Read the model definition and answer for the solid it produces. Units are mm, in the model's axes. Face numbers are marked on the shaded views. A direction names the side the tool comes from. Coordinates: 2 decimals unless noted, no trailing zeros. Loops run counter-clockwise (first coordinate to the right, second up) from the corner with the lowest first, then second, coordinate; pieces in that order, holes last. Notation, with made-up numbers: M 49,14.5 L 79,14.5 A4 cw 79,20.5 Z; hole C 22,75 d3. An arc over 180 degrees is marked long. One line per item, written item: value. Start each with the question number.
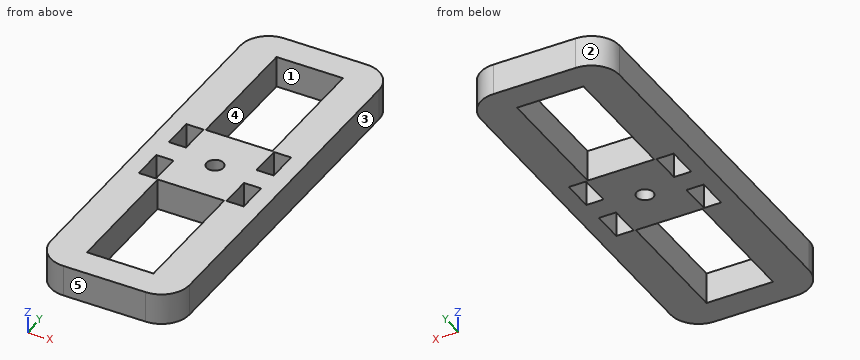
```python
from build123d import *

# Parameters (mm, degrees)
SKETCH1_W           = 3.055
SKETCH1_H           = 5.575
SKETCH1_W_2         = 11.81
SKETCH1_H_2         = 22.57
SKETCH1_R           = 1.475
BOSS_EXTRUDE1_DEPTH = 5.58


with BuildPart() as part:
    # Sketch1 → Boss-Extrude1 (new body)
    with BuildSketch(Plane.XY):
        with BuildLine():
            Line((708.390729089, 432.709671907), (715.695729089, 432.709671907))
            Line((715.695729089, 432.709671907), (723.000729089, 432.709671907))
            ThreePointArc((723.000729089, 432.709671907), (726.536262995, 434.174138001), (728.000729089, 437.709671907))
            Line((728.000729089, 437.709671907), (728.000729089, 498.199671907))
            ThreePointArc((728.000729089, 498.199671907), (726.536262995, 501.735205812), (723.000729089, 503.199671907))
            Line((723.000729089, 503.199671907), (715.695729089, 503.199671907))
            Line((715.695729089, 503.199671907), (708.390729089, 503.199671907))
            ThreePointArc((708.390729089, 503.199671907), (704.855195183, 501.735205812), (703.390729089, 498.199671907))
            Line((703.390729089, 498.199671907), (703.390729089, 437.709671907))
            ThreePointArc((703.390729089, 437.709671907), (704.855195183, 434.174138001), (708.390729089, 432.709671907))
        make_face()
        with Locations((707.918229089, 463.167171907)):
            Rectangle(SKETCH1_W, SKETCH1_H, mode=Mode.SUBTRACT)
        with Locations((715.695729089, 448.994671907)):
            Rectangle(SKETCH1_W_2, SKETCH1_H_2, mode=Mode.SUBTRACT)
        with Locations((715.695729089, 467.954671907)):
            Circle(SKETCH1_R, mode=Mode.SUBTRACT)
        with Locations((723.473229089, 463.167171907)):
            Rectangle(SKETCH1_W, SKETCH1_H, mode=Mode.SUBTRACT)
        with Locations((707.918229089, 472.742171907)):
            Rectangle(SKETCH1_W, SKETCH1_H, mode=Mode.SUBTRACT)
        with Locations((723.473229089, 472.742171907)):
            Rectangle(SKETCH1_W, SKETCH1_H, mode=Mode.SUBTRACT)
        with Locations((715.695729089, 486.914671907)):
            Rectangle(SKETCH1_W_2, SKETCH1_H_2, mode=Mode.SUBTRACT)
    extrude(amount=BOSS_EXTRUDE1_DEPTH)


solid = part.part
```
1) Flat-ended cylindrical pins translate along their axes: pin 1 (1.5 mm diameter, centred on x = 724, z = 4, fed in from -Y); pin 2 (2 mm diameter, centred on x = 719, y = 453.5, fed in from -Z); pin 3 (1.5 mm diameter, centred on x = 724.5, z = 2, fed in from +Y); pin 4 (0.9 mm diameter, centred on x = 707.5, z = 3, fed in from +Y). Find the tip coordinate at first contact, or state that the pin passes through.
2) Section C-C (x = 715) is taken. Determine the outline of the cut face in (y, z), then the cut area to 3 significant figures.
3) A tool of negligible diameter and unlimited length cuts with its end or side. For the marked faces 1 and 2, from which of +Z, -Z, +X, -X, +Y, -Y can it reach the whole face along a straight path? Write none if from no direction.
4) Consider line 1 along Y through (x, z) = (708.75, 4.1); line 2 along Y through (x, z) = (710.25, 2.05); line 3 along X through (y, z) = (472, 3.8). Determine where each line is inside the solid, lowest interval first.
5) Section B-B (y = 478) is taken. Determine the outline of the cut face in (x, z), then the cut area to 3 significant figures.
6) For a pull along Y with two mould halves and no side action, classify the marked faces 3, 4 and 5 as released by +Y, released by -Y, zero draft, split by the parting line, or undercut.
7) Section D-D (x = 718.5) is taken. Determine the outline of the cut face in (y, z).
8) Section A-A (y = 462.5) is taken. Determine the outline of the cut face in (x, z), then the cut area to 3 significant figures.
Results found:
1. pin 1: stops at y = 432.72
1. pin 2: passes through
1. pin 3: stops at y = 503.14
1. pin 4: stops at y = 503.18
2. outline: M 432.71,0 L 437.71,0 L 437.71,5.58 L 432.71,5.58 Z; M 460.28,0 L 466.65,0 L 466.65,5.58 L 460.28,5.58 Z; M 469.26,0 L 475.63,0 L 475.63,5.58 L 469.26,5.58 Z; M 498.2,0 L 503.2,0 L 503.2,5.58 L 498.2,5.58 Z
2. area: 127 mm²
3. face 1: +Z, -Z
3. face 2: +Z, -Z, -X, +Y
4. line 1: y = 432.71 to 460.38, 465.95 to 469.95, 475.53 to 503.2
4. line 2: y = 432.71 to 437.71, 460.28 to 475.63, 498.2 to 503.2
4. line 3: x = 703.39 to 706.39, 709.45 to 721.95, 725 to 728
5. outline: M 703.39,0 L 709.79,0 L 709.79,5.58 L 703.39,5.58 Z; M 721.6,0 L 728,0 L 728,5.58 L 721.6,5.58 Z
5. area: 71.4 mm²
6. face 3: zero draft
6. face 4: undercut
6. face 5: released by -Y
7. outline: M 432.71,0 L 437.71,0 L 437.71,5.58 L 432.71,5.58 Z; M 460.28,0 L 475.63,0 L 475.63,5.58 L 460.28,5.58 Z; M 498.2,0 L 503.2,0 L 503.2,5.58 L 498.2,5.58 Z
8. outline: M 703.39,0 L 706.39,0 L 706.39,5.58 L 703.39,5.58 Z; M 709.45,0 L 721.95,0 L 721.95,5.58 L 709.45,5.58 Z; M 725,0 L 728,0 L 728,5.58 L 725,5.58 Z
8. area: 103 mm²
